```python
from build123d import *

# Parameters (mm, degrees)
BOSS_EXTRUDE1_DEPTH = 12
SKETCH4_R           = 2
CUT_EXTRUDE2_DEPTH  = 100.249994256
FILLET2_R           = 8


with BuildPart() as part:
    # Sketch1 → Boss-Extrude1 (new body)
    with BuildSketch(Plane.XY):
        with BuildLine():
            Line((61.423127431, 25), (55.463282958, 25))
            Line((55.463282958, 25), (10.60599556, -12.639733311))
            Line((10.60599556, -12.639733311), (10.60599556, -24.566634818))
            ThreePointArc((10.60599556, -24.566634818), (24.944333721, -22.584404279), (38.973425347, -19.020450397))
            ThreePointArc((38.973425347, -19.020450397), (58.129824232, -14.452456897), (77.737673628, -12.617674908))
            Line((77.737673628, -12.617674908), (95.297226402, 2.116539348))
            Line((95.297226402, 2.116539348), (87.463282958, 23.640122064))
            ThreePointArc((87.463282958, 23.640122064), (74.460947109, 24.659799043), (61.423127431, 25))
        make_face()
    extrude(amount=BOSS_EXTRUDE1_DEPTH)

    # Sketch4 → Cut-Extrude2 (cut, through all)
    with BuildSketch(Plane.XY.offset(12)):
        with Locations((30.070163865, -10.944644586)):
            Circle(SKETCH4_R)
        with Locations((83.953508951, 13.296929528)):
            Circle(SKETCH4_R)
        with Locations((60, 0)):
            Circle(SKETCH4_R)
    extrude(amount=-CUT_EXTRUDE2_DEPTH, mode=Mode.SUBTRACT)

    # Fillet2
    # the kernel refuses this fillet: 8 mm, written as the material it takes off along each edge
    with BuildSketch(Plane(origin=(77.737673628, -12.617674908, -6.911835491), x_dir=(0.7660444431189745, 0.6427876096865436, 0), z_dir=(0, 0, 1))) as fillet2_piece_1:
        with BuildLine():
            CenterArc((2.764734197, 8), FILLET2_R, 232.413146156, 37.586853844)
            ThreePointArc((-2.114972699, 1.660563068), (-1.053499463, 0.835359424), (0, 0))
            Line((0, 0), (2.764734197, 0))
        make_face()
    extrude(amount=25.823670983, mode=Mode.SUBTRACT)
    with BuildSketch(Plane(origin=(10.60599556, -24.566634818, -23.209901988), x_dir=(0, 1, 0), z_dir=(0, 0, 1))) as fillet2_piece_2:
        with BuildLine():
            CenterArc((8.993765029, -8), FILLET2_R, 90, 98.772306206)
            ThreePointArc((1.087347338, -9.220065283), (0.461340951, -4.619742362), (0, 0))
            Line((0, 0), (8.993765029, 0))
        make_face()
    extrude(amount=58.419803977, mode=Mode.SUBTRACT)
    with BuildSketch(Plane(origin=(10.60599556, -12.639733311, -9.326153163), x_dir=(0.7660444431189766, 0.6427876096865411, 0), z_dir=(0, 0, 1))) as fillet2_piece_3:
        with BuildLine():
            CenterArc((FILLET2_R * 0.466307658155, -FILLET2_R), FILLET2_R, 90, 50)
            Line((-FILLET2_R * 0.299736784964, -FILLET2_R * 0.357212390313), (0, 0))
            Line((0, 0), (FILLET2_R * 0.466307658155, 0))
        make_face()
    extrude(amount=30.652306326, mode=Mode.SUBTRACT)
    with BuildSketch(Plane(origin=(95.297226402, 2.116539348, -14.004150764), x_dir=(-0.34202014332566766, 0.9396926207859088, 0), z_dir=(0, 0, 1))) as fillet2_piece_4:
        with BuildLine():
            CenterArc((FILLET2_R * 0.70020753821, FILLET2_R), FILLET2_R, 200, 70)
            Line((-FILLET2_R * 0.239485082576, FILLET2_R * 0.657979856674), (0, 0))
            Line((0, 0), (FILLET2_R * 0.70020753821, 0))
        make_face()
    extrude(amount=40.008301528, mode=Mode.SUBTRACT)
    with BuildSketch(Plane(origin=(87.463282958, 23.640122064, -12.852127182), x_dir=(-0.9955788661369174, 0.0939293420690782, 0), z_dir=(0, 0, 1))) as fillet2_piece_5:
        with BuildLine():
            CenterArc((5.058597259, 7.999577135), FILLET2_R, 205.389700078, 65.199408418)
            Line((-2.168701836, 4.569395246), (0, 0))
            ThreePointArc((0, 0), (2.570425436, -0.013214523), (5.140850873, 0))
        make_face()
    extrude(amount=37.704254365, mode=Mode.SUBTRACT)
    with BuildSketch(Plane(origin=(55.463282958, 25, -7.279404685), x_dir=(1, 0, 0), z_dir=(0, 0, 1))) as fillet2_piece_6:
        with BuildLine():
            CenterArc((FILLET2_R * 0.363970234266, -FILLET2_R), FILLET2_R, 90, 40)
            Line((-FILLET2_R * 0.27881737542, -FILLET2_R * 0.233955556881), (0, 0))
            Line((0, 0), (FILLET2_R * 0.363970234266, 0))
        make_face()
    extrude(amount=26.558809371, mode=Mode.SUBTRACT)


solid = part.part
```
Input: part model. Units: mm. Frame: model coordinates. Give positions to 0.01 mm unless a question says otherwise; leave off trailing zeros. Loops run counter-clockwise (first coordinate to the right, second up) from the corner with the lowest first, then second, coordinate; pieces in that order, holes last.
1) Section query B-B on z = 7.25. Return the cut outline in (x, y), and give its area (3 significant figures).
A:
outline: (10.62, -15.97) arc R8 ccw to (19.83, -23.48) arc R130 ccw to (38.97, -19.02) arc R140 cw to (75.05, -12.71) arc R8 ccw to (79.86, -10.84) - (91.01, -1.48) arc R8 ccw to (93.38, 7.38) - (89.19, 18.89) arc R8 ccw to (82.35, 24.12) arc R250 ccw to (61.42, 25) - (58.38, 25) arc R8 ccw to (53.23, 23.13) - (13.46, -10.24) arc R8 ccw to start; hole circle Ø4 at (30.07, -10.94); hole circle Ø4 at (60, 0); hole circle Ø4 at (83.95, 13.3)
area: 2,400 mm2
2) Line query: L1, parallel to X at y = -1, z = 11; L2, parallel to Y at x = 83, z = 7.25 (3 decimals); L3, parallel to X at y = -6, z = 10.75. Output: solid intervals per line, ascending.
A:
L1: x = 24.48 to 58.27, 61.73 to 91.53
L2: y = -8.202 to 11.539, 15.055 to 24.041
L3: x = 18.52 to 85.62
3) Mould query, pull axis X, two halves, no side actions, for faces 1 (the cylindrical face through (58, 0, 6)), 2 (the cylindrical face through (93.573, 2.508, 5.916)), 3 (the flat face through (52, 1, 12)). Classes: released by +X, released by -X, zero draft, split by the parting line, or undercut.
A:
face 1: undercut
face 2: released by +X
face 3: zero draft
4) Section query A-A on x = 60. Return the cut outline in (y, z), and give its area (3 significant figures).
A:
outline: (-14.16, 0) - (-2, 0) - (-2, 12) - (-14.16, 12) - close; (2, 0) - (25, 0) - (25, 12) - (2, 12) - close
area: 422 mm2
5) Section query C-C on y = 0. Return the cut outline in (x, z), and give its area (4 significant figures).
A:
outline: (25.67, 0) - (58, 0) - (58, 12) - (25.67, 12) - close; (62, 0) - (92.38, 0) - (92.38, 12) - (62, 12) - close
area: 752.5 mm2
6) Contact query for flat-ended pins moving along their axis: pin 1 (2 mm diameter, centred on y = -5.5, z = 3.5, fed in from -X); pin 2 (5 mm diameter, centred on x = 45, z = 9.5, fed in from +Y). Output: stop coordinate, or through.
A:
pin 1: stops at x = 17.92
pin 2: stops at y = 18.32
7) Section query D-D on x = 40.5. Return the cut outline in (y, z).
A:
outline: (-18.55, 0) - (12.44, 0) - (12.44, 12) - (-18.55, 12) - close
